Model file for the job. Use its own axes, mm. Face numbers are marked on the shaded views. A direction names the side the tool comes from. Round coordinates to 2 decimals unless told otherwise and drop trailing zeros. Loops run counter-clockwise (first coordinate to the right, second up) from the corner with the lowest first, then second, coordinate; pieces in that order, holes last. Notation, with made-up numbers: M 7,75 L 50,75 A15 cw 50,93 Z; hole C 19,83 d7. An arc over 180 degrees is marked long. Use a Markdown table: item, result. Add a question column.
Item 1: Tool access for the marked faces 1 and 2: list every direction of +Z, -Z, +X, -X, +Y, -Y with a clear straight run to the whole face (end or side of a thin tool).
Item 2: Saw through at B-B on y = 6. Write the cut outline in (x, z).
Item 3: Saw through at A-A on x = 30. Write the cut outline in (y, z).
Item 4: Saw through at D-D on x = 48.25. Write the cut outline in (y, z).
Item 5: Saw through at C-C on z = -15.5. Write the cut outline in (x, y).
Item 6: Wall check: L1, parallel to X at y = 17, z = -30; L2, parallel to Z at x = 48, y = 15; L3, parallel to Y at x = 6, z = -48. Give the ranges that are in metal, low to high. Write a range as from..to.
Item 7: Two-plate mould, pull along Z, no slides. Class the marked faces 3, 4 and 5: +Z half, -Z half, draft (parallel to the pull), parting line (faces both ways), or undercut.
Item 8: Pin check, flat tips, straight feed: P1, Ø1.1, axis at y = 15, z = -48, coming from the -X side; P2, Ø1.5, axis at x = 7, y = 11.5, coming from the -Z side; P3, Ø1.5, axis at y = 16, z = -29, coming from the -X side. Stop position of each tip, or through.
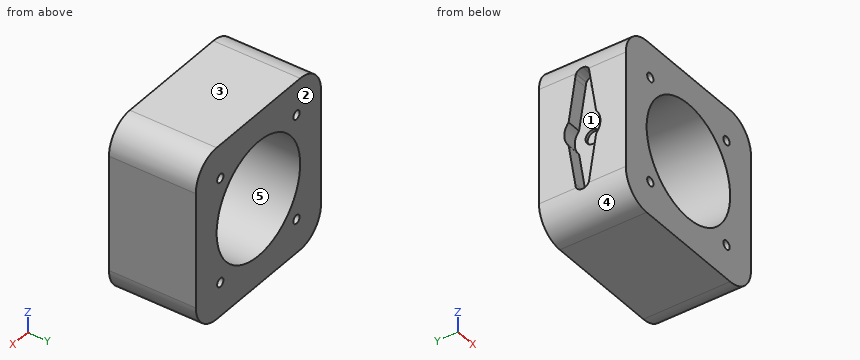
```python
from build123d import *

# Parameters (mm, degrees)
SKETCH1_W           = 60
SKETCH1_H           = 60
SKETCH1_R           = 20
SKETCH1_R_2         = 1.5
BOSS_EXTRUDE1_DEPTH = 30
FILLET1_R           = 10
SKETCH2_R           = 6.25
CUT_EXTRUDE1_DEPTH  = 5
SKETCH3_R           = 2.5
CUT_EXTRUDE4_DEPTH  = 1
SKETCH4_R           = 0.5
CUT_EXTRUDE5_DEPTH  = 2


with BuildPart() as part:
    # Sketch1 → Boss-Extrude1 (new body)
    with BuildSketch(Plane(origin=(0, 0, 0), x_dir=(1, 0, 0), z_dir=(0, 1, 0))):
        with Locations((30, 30)):
            Rectangle(SKETCH1_W, SKETCH1_H)
        with Locations(Location((30, 30, 0), (0, 0, 270))):
            Circle(SKETCH1_R, mode=Mode.SUBTRACT)
        with Locations(Location((48.25, 48.25, 0), (0, 0, 270))):
            Circle(SKETCH1_R_2, mode=Mode.SUBTRACT)
        with Locations(Location((11.75, 48.25, 0), (0, 0, 270))):
            Circle(SKETCH1_R_2, mode=Mode.SUBTRACT)
        with Locations(Location((11.75, 11.75, 0), (0, 0, 270))):
            Circle(SKETCH1_R_2, mode=Mode.SUBTRACT)
        with Locations(Location((48.25, 11.75, 0), (0, 0, 270))):
            Circle(SKETCH1_R_2, mode=Mode.SUBTRACT)
    extrude(amount=BOSS_EXTRUDE1_DEPTH)

    # Fillet1
    fillet1_edges = [part.edges().sort_by_distance(p)[0] for p in [
        (0, 15, -60),
        (60, 15, -60),
        (60, 15, 0),
        (0, 15, 0),
    ]]
    fillet(fillet1_edges, radius=FILLET1_R)

    # Sketch2 → Cut-Extrude1 (cut)
    with BuildSketch(Plane.ZY):
        with BuildLine():
            Line((-34.062019202, 19.75), (-48.409222121, 17.476665185))
            ThreePointArc((-48.409222121, 17.476665185), (-46.865597615, 16.642871769), (-46.25, 15))
            ThreePointArc((-46.25, 15), (-46.865597615, 13.357128231), (-48.409222121, 12.523334815))
            Line((-48.409222121, 12.523334815), (-34.062019202, 10.25))
            ThreePointArc((-34.062019202, 10.25), (-36.25, 15), (-34.062019202, 19.75))
        make_face()
        with Locations((-30, 15)):
            Circle(SKETCH2_R)
        with BuildLine():
            Line((-11.590777879, 17.476665185), (-25.937980798, 19.75))
            ThreePointArc((-25.937980798, 19.75), (-24.323287923, 17.614849899), (-23.75, 15))
            ThreePointArc((-23.75, 15), (-24.323287923, 12.385150101), (-25.937980798, 10.25))
            Line((-25.937980798, 10.25), (-11.590777879, 12.523334815))
            ThreePointArc((-11.590777879, 12.523334815), (-13.75, 15), (-11.590777879, 17.476665185))
        make_face()
        with BuildLine():
            Line((-10.160275264, 17.25), (-11.590777879, 17.476665185))
            ThreePointArc((-11.590777879, 17.476665185), (-13.75, 15), (-11.590777879, 12.523334815))
            Line((-11.590777879, 12.523334815), (-10.160275264, 12.75))
            ThreePointArc((-10.160275264, 12.75), (-10.079367047, 12.791014149), (-10, 12.834936491))
            Line((-10, 12.834936491), (-10, 17.165063509))
            ThreePointArc((-10, 17.165063509), (-10.079367047, 17.208985851), (-10.160275264, 17.25))
        make_face()
        with BuildLine():
            ThreePointArc((-8.75, 15), (-9.084936491, 16.25), (-10, 17.165063509))
            Line((-10, 17.165063509), (-10, 12.834936491))
            ThreePointArc((-10, 12.834936491), (-9.084936491, 13.75), (-8.75, 15))
        make_face()
        with BuildLine():
            Line((-48.409222121, 17.476665185), (-49.839724736, 17.25))
            ThreePointArc((-49.839724736, 17.25), (-49.920632953, 17.208985851), (-50, 17.165063509))
            Line((-50, 17.165063509), (-50, 12.834936491))
            ThreePointArc((-50, 12.834936491), (-49.920632953, 12.791014149), (-49.839724736, 12.75))
            Line((-49.839724736, 12.75), (-48.409222121, 12.523334815))
            ThreePointArc((-48.409222121, 12.523334815), (-46.865597615, 13.357128231), (-46.25, 15))
            ThreePointArc((-46.25, 15), (-46.865597615, 16.642871769), (-48.409222121, 17.476665185))
        make_face()
        with BuildLine():
            Line((-50, 12.834936491), (-50, 17.165063509))
            ThreePointArc((-50, 17.165063509), (-51.25, 15), (-50, 12.834936491))
        make_face()
    extrude(amount=-CUT_EXTRUDE1_DEPTH, mode=Mode.SUBTRACT)

    # Sketch3 → Cut-Extrude4 (cut)
    with BuildSketch(Plane.ZY.offset(-5)):
        with Locations((-30, 15)):
            Circle(SKETCH3_R)
    extrude(amount=-CUT_EXTRUDE4_DEPTH, mode=Mode.SUBTRACT)

    # Sketch4 → Cut-Extrude5 (cut)
    with BuildSketch(Plane.ZY.offset(-5)):
        with Locations((-12, 15)):
            Circle(SKETCH4_R)
        with Locations((-48, 15)):
            Circle(SKETCH4_R)
    extrude(amount=-CUT_EXTRUDE5_DEPTH, mode=Mode.SUBTRACT)


solid = part.part
```
Entries:
| question | item | result |
|---|---|---|
| 1 | face 1 | -X |
| 1 | face 2 | +Z, -Z, +X, -X, +Y |
| 2 | outline | M 0,-50 A10 ccw 10,-60 L 50,-60 A10 ccw 60,-50 L 60,-10 A10 ccw 50,0 L 10,0 A10 ccw 0,-10 Z; hole C 30,-30 d40; hole C 11.75,-48.25 d3; hole C 11.75,-11.75 d3; hole C 48.25,-48.25 d3; hole C 48.25,-11.75 d3 |
| 3 | outline | M 0,-60 L 30,-60 L 30,-50 L 0,-50 Z; M 0,-10 L 30,-10 L 30,0 L 0,0 Z |
| 4 | outline | M 0,-60 L 30,-60 L 30,-49.75 L 0,-49.75 Z; M 0,-46.75 L 30,-46.75 L 30,-38.18 L 0,-38.18 Z; M 0,-21.82 L 30,-21.82 L 30,-13.25 L 0,-13.25 Z; M 0,-10.25 L 30,-10.25 L 30,0 L 0,0 Z |
| 5 | outline | M 0,0 L 16.23,0 L 16.23,30 L 0,30 L 0,18.1 L 5,18.1 L 5,11.9 L 0,11.9 Z; M 43.77,0 L 60,0 L 60,30 L 43.77,30 Z |
| 6 | L1 | 6..10, 50..60 |
| 6 | L2 | -60..-49.73, -46.77..-38.72, -21.28..-13.23, -10.27..0 |
| 6 | L3 | 0..14.5, 15.5..30 |
| 7 | face 3 | +Z half |
| 7 | face 4 | -Z half |
| 7 | face 5 | undercut |
| 8 | P1 | x = 5 |
| 8 | P2 | z = -59.74 |
| 8 | P3 | x = 6 |
